```python
from build123d import *

# Parameters (mm, degrees)
SKETCH_1_R          = 1.6
EXTRUDE_1_DEPTH     = 3
EXTRUDE_2_DEPTH     = 50
SKETCH_2_R          = 1.6
SKETCH_2_W          = 4
SKETCH_2_H          = 21
CUT_EXTRUDE_1_DEPTH = 6
SKETCH_3_W          = 7
SKETCH_3_H          = 16.993149035
CUT_EXTRUDE_5_DEPTH = 1.8


with BuildPart() as part:
    # 草图1 → 凸台-拉伸1 (new body)
    with BuildSketch(Plane(origin=(0, 0, 0), x_dir=(1, 0, 0), z_dir=(0, 1, 0))):
        Polygon((-10, 0), (0, 0), (10, 0), (15, 0), (15, 25), (10, 25), (-15, 25), (-15, 0), align=None)
        with Locations((-10, 5)):
            Circle(SKETCH_1_R, mode=Mode.SUBTRACT)
        with BuildLine():
            ThreePointArc((11.6, 5), (8.86862915, 3.86862915), (10, 6.6))
            ThreePointArc((10, 6.6), (11.13137085, 6.13137085), (11.6, 5))
        make_face(mode=Mode.SUBTRACT)
    extrude(amount=EXTRUDE_1_DEPTH)

    # 草图1<3> → 凸台-拉伸2 (add)
    with BuildSketch(Plane(origin=(0, 0, 0), x_dir=(1, 0, 0), z_dir=(0, 1, 0))):
        Polygon((10, 25), (15, 25), (15, 30), (-15, 30), (-15, 25), align=None)
    extrude(amount=EXTRUDE_2_DEPTH)

    # 草图2 → 切除-拉伸1 (cut, through all)
    with BuildSketch(Plane.XY.offset(-25)):
        with Locations((0, 47.5)):
            Circle(SKETCH_2_R)
        with Locations((0, 26.5)):
            Circle(SKETCH_2_R)
        with Locations((6, 37)):
            Rectangle(SKETCH_2_W, SKETCH_2_H)
        with Locations((-5.879917392, 37)):
            Rectangle(SKETCH_2_W, SKETCH_2_H)
    extrude(amount=-CUT_EXTRUDE_1_DEPTH, mode=Mode.SUBTRACT)

    # 草图3 → 切除-拉伸5 (cut)
    with BuildSketch(Plane.XY.offset(-25)):
        with Locations((0, 37.216442025)):
            Rectangle(SKETCH_3_W, SKETCH_3_H)
    extrude(amount=-CUT_EXTRUDE_5_DEPTH, mode=Mode.SUBTRACT)


solid = part.part
```
CAD build for the part. Positions are in the model's coordinates, mm. A direction names the side the tool comes from. Give positions to 0.01 mm unless a question says otherwise; leave off trailing zeros. Order: outer loops, then holes, each group sorted by start corner. A loop starts at its lowest first (then second) coordinate and runs counter-clockwise, first axis right, second up.
(1) Saw through at C-C, the plane y = 4. Give the cut face in (x, z).
(2) Saw through at A-A, the plane x = -10. Give the cut face in (y, z).
(3) Saw through at D-D, the plane z = -9.5. Give the cut face in (x, y), then the cut area to 3 significant figures.
(4) Saw through at B-B, the plane x = 0. Give the cut face in (y, z), then the cut area to 3 significant figures.
(5) Drill centre lines: L1, parallel to Y at x = 0, z = -26.4; L2, parallel to X at y = 1.5, z = -5; L3, parallel to Y at x = 0, z = -27.35. Where is each one in solid material? Low to high.
(6) Flat gauge pins, fed straight in: pin 1 (4 mm diameter, centred on x = 0, y = 26.5, fed in from +Z); pin 2 (2 mm diameter, centred on x = -0.5, y = 33, fed in from +Z); pin 3 (2 mm diameter, centred on x = 5, z = -15, fed in from -Y). Where does each tip first touch, or does it go through?
(7) Tool access for faces 1 (the flat face through (15, 17, -26)), 2 (the flat face through (-7.88, 37, -27)), 3 (the flat face through (0, 45.713, -26)): list every direction of +Z, -Z, +X, -X, +Y, -Y with a clear straight run to the whole face (end or side of a thin tool).
(8) Mould opens along X. For faces 4 (the flat face through (8, 37, -27)), 5 (the flat face through (0, 50, -28)), 6 (the flat face through (-3.5, 37, -26)), 7 (the flat face through (-15, 17, -26)) say: released by +X, released by -X, zero draft, split by the parting line, or undercut.
Results found:
1. outline: (-15, -30) - (15, -30) - (15, -25) - (-15, -25) - close
2. outline: (0, -30) - (50, -30) - (50, -25) - (3, -25) - (3, -6.6) - (0, -6.6) - close; (0, -3.4) - (3, -3.4) - (3, 0) - (0, 0) - close
3. outline: (-15, 0) - (15, 0) - (15, 3) - (-15, 3) - close
3. area: 90.0 mm2
4. outline: (0, -30) - (24.9, -30) - (24.9, -25) - (3, -25) - (3, 0) - (0, 0) - close; (28.1, -30) - (45.9, -30) - (45.9, -25) - (45.71, -25) - (45.71, -26.8) - (28.72, -26.8) - (28.72, -25) - (28.1, -25) - close; (49.1, -30) - (50, -30) - (50, -25) - (49.1, -25) - close
4. area: 262 mm2
5. L1: y = 0 to 24.9, 28.1 to 28.72, 45.71 to 45.9, 49.1 to 50
5. L2: x = -15 to -11.6, -8.4 to 8.4, 11.6 to 15
5. L3: y = 0 to 24.9, 28.1 to 45.9, 49.1 to 50
6. pin 1: stops at z = -25
6. pin 2: stops at z = -26.8
6. pin 3: stops at y = 0
7. face 1: +Z, -Z, +X, +Y, -Y
7. face 2: +Z, -Z
7. face 3: +Z
8. face 4: undercut
8. face 5: zero draft
8. face 6: undercut
8. face 7: released by -X
